CAD build for the part. Positions are in the model's coordinates, mm. Give positions to 0.01 mm unless a question says otherwise; leave off trailing zeros. Loops run counter-clockwise (first coordinate to the right, second up) from the corner with the lowest first, then second, coordinate; pieces in that order, holes last. Notation, with made-up numbers: (14, 28) -> (19, 28) arc R15 cw to (19, 51) -> close; hole circle Ø2 at (62.5, 30.5). An arc over 180 degrees is marked (long way). Use one line per item in the form item = value.
```python
from build123d import *

# Parameters (mm, degrees)
F0_R     = 50
F1_DEPTH = 10
F2_R     = 125
F2_R_2   = 40.44952
F3_DEPTH = 10
F5_DEPTH = 25


with BuildPart() as f1:
    # F0 (on Top) → F1 (new body)
    with BuildSketch(Plane.XY):
        Circle(F0_R)
        Polygon((-10, 30), (0, 30), (10, 30), (10, 10), (30, 10), (30, 0), (30, -10), (10, -10), (10, -30), (0, -30), (-10, -30), (-10, -10), (-30, -10), (-30, 0), (-30, 10), (-10, 10), align=None, mode=Mode.SUBTRACT)
    extrude(amount=F1_DEPTH)

    # F2 (on face) → F3 (join)
    with BuildSketch(Plane.XY.offset(10)):
        Circle(F2_R)
        Circle(F2_R_2, mode=Mode.SUBTRACT)
    extrude(amount=-F3_DEPTH)

    # F4 (on face) → F5 (cut)
    with BuildSketch(Plane.XY.offset(10)):
        with BuildLine():
            Line((0, 116.456337), (0, 104.802647))
            ThreePointArc((0, 104.802647), (9.134153, 104.403842), (18.198789, 103.21046))
            Line((18.198789, 103.21046), (20.222431, 114.687104))
            ThreePointArc((20.222431, 114.687104), (10.149839, 116.013186), (0, 116.456337))
        make_face()
        with BuildLine():
            ThreePointArc((-35.844616, 98.482274), (-27.124921, 101.231584), (-18.198789, 103.21046))
            Line((-18.198789, 103.21046), (-20.222431, 114.687104))
            ThreePointArc((-20.222431, 114.687104), (-30.141118, 112.488184), (-39.830413, 109.433161))
            Line((-39.830413, 109.433161), (-35.844616, 98.482274))
        make_face()
        with BuildLine():
            ThreePointArc((-67.365843, 80.283486), (-60.112329, 85.849303), (-52.401324, 90.761755))
            Line((-52.401324, 90.761755), (-58.228169, 100.854147))
            ThreePointArc((-58.228169, 100.854147), (-66.796611, 95.395447), (-74.856691, 89.21073))
            Line((-74.856691, 89.21073), (-67.365843, 80.283486))
        make_face()
        with BuildLine():
            ThreePointArc((-90.761755, 52.401324), (-85.849303, 60.112329), (-80.283486, 67.365843))
            Line((-80.283486, 67.365843), (-89.21073, 74.856691))
            ThreePointArc((-89.21073, 74.856691), (-95.395447, 66.796611), (-100.854147, 58.228169))
            Line((-100.854147, 58.228169), (-90.761755, 52.401324))
        make_face()
        with BuildLine():
            ThreePointArc((-103.21046, 18.198789), (-101.231584, 27.124921), (-98.482274, 35.844616))
            Line((-98.482274, 35.844616), (-109.433161, 39.830413))
            ThreePointArc((-109.433161, 39.830413), (-112.488184, 30.141118), (-114.687104, 20.222431))
            Line((-114.687104, 20.222431), (-103.21046, 18.198789))
        make_face()
        with BuildLine():
            ThreePointArc((-103.21046, -18.198789), (-104.403842, -9.134153), (-104.802647, 0))
            Line((-104.802647, 0), (-116.456337, 0))
            ThreePointArc((-116.456337, 0), (-116.013186, -10.149839), (-114.687104, -20.222431))
            Line((-114.687104, -20.222431), (-103.21046, -18.198789))
        make_face()
        with BuildLine():
            ThreePointArc((-90.761755, -52.401324), (-94.983455, -44.291513), (-98.482274, -35.844616))
            Line((-98.482274, -35.844616), (-109.433161, -39.830413))
            ThreePointArc((-109.433161, -39.830413), (-105.545285, -49.216575), (-100.854147, -58.228169))
            Line((-100.854147, -58.228169), (-90.761755, -52.401324))
        make_face()
        with BuildLine():
            ThreePointArc((-67.365843, -80.283486), (-74.106663, -74.106663), (-80.283486, -67.365843))
            Line((-80.283486, -67.365843), (-89.21073, -74.856691))
            ThreePointArc((-89.21073, -74.856691), (-82.347066, -82.347066), (-74.856691, -89.21073))
            Line((-74.856691, -89.21073), (-67.365843, -80.283486))
        make_face()
        with BuildLine():
            ThreePointArc((-35.844616, -98.482274), (-44.291513, -94.983455), (-52.401324, -90.761755))
            Line((-52.401324, -90.761755), (-58.228169, -100.854147))
            ThreePointArc((-58.228169, -100.854147), (-49.216575, -105.545285), (-39.830413, -109.433161))
            Line((-39.830413, -109.433161), (-35.844616, -98.482274))
        make_face()
        with BuildLine():
            ThreePointArc((0, -104.802647), (-9.134153, -104.403842), (-18.198789, -103.21046))
            Line((-18.198789, -103.21046), (-20.222431, -114.687104))
            ThreePointArc((-20.222431, -114.687104), (-10.149839, -116.013186), (0, -116.456337))
            Line((0, -116.456337), (0, -104.802647))
        make_face()
        with BuildLine():
            ThreePointArc((35.844616, -98.482274), (27.124921, -101.231584), (18.198789, -103.21046))
            Line((18.198789, -103.21046), (20.222431, -114.687104))
            ThreePointArc((20.222431, -114.687104), (30.141118, -112.488184), (39.830413, -109.433161))
            Line((39.830413, -109.433161), (35.844616, -98.482274))
        make_face()
        with BuildLine():
            ThreePointArc((67.365843, -80.283486), (60.112329, -85.849303), (52.401324, -90.761755))
            Line((52.401324, -90.761755), (58.228169, -100.854147))
            ThreePointArc((58.228169, -100.854147), (66.796611, -95.395447), (74.856691, -89.21073))
            Line((74.856691, -89.21073), (67.365843, -80.283486))
        make_face()
        with BuildLine():
            ThreePointArc((90.761755, -52.401324), (85.849303, -60.112329), (80.283486, -67.365843))
            Line((80.283486, -67.365843), (89.21073, -74.856691))
            ThreePointArc((89.21073, -74.856691), (95.395447, -66.796611), (100.854147, -58.228169))
            Line((100.854147, -58.228169), (90.761755, -52.401324))
        make_face()
        with BuildLine():
            ThreePointArc((103.21046, -18.198789), (101.231584, -27.124921), (98.482274, -35.844616))
            Line((98.482274, -35.844616), (109.433161, -39.830413))
            ThreePointArc((109.433161, -39.830413), (112.488184, -30.141118), (114.687104, -20.222431))
            Line((114.687104, -20.222431), (103.21046, -18.198789))
        make_face()
        with BuildLine():
            ThreePointArc((103.21046, 18.198789), (104.403842, 9.134153), (104.802647, 0))
            Line((104.802647, 0), (116.456337, 0))
            ThreePointArc((116.456337, 0), (116.013186, 10.149839), (114.687104, 20.222431))
            Line((114.687104, 20.222431), (103.21046, 18.198789))
        make_face()
        with BuildLine():
            ThreePointArc((90.761755, 52.401324), (94.983455, 44.291513), (98.482274, 35.844616))
            Line((98.482274, 35.844616), (109.433161, 39.830413))
            ThreePointArc((109.433161, 39.830413), (105.545285, 49.216575), (100.854147, 58.228169))
            Line((100.854147, 58.228169), (90.761755, 52.401324))
        make_face()
        with BuildLine():
            ThreePointArc((67.365843, 80.283486), (74.106663, 74.106663), (80.283486, 67.365843))
            Line((80.283486, 67.365843), (89.21073, 74.856691))
            ThreePointArc((89.21073, 74.856691), (82.347066, 82.347066), (74.856691, 89.21073))
            Line((74.856691, 89.21073), (67.365843, 80.283486))
        make_face()
        with BuildLine():
            ThreePointArc((35.844616, 98.482274), (44.291513, 94.983455), (52.401324, 90.761755))
            Line((52.401324, 90.761755), (58.228169, 100.854147))
            ThreePointArc((58.228169, 100.854147), (49.216575, 105.545285), (39.830413, 109.433161))
            Line((39.830413, 109.433161), (35.844616, 98.482274))
        make_face()
    extrude(amount=-F5_DEPTH, mode=Mode.SUBTRACT)


solid = f1.part
```
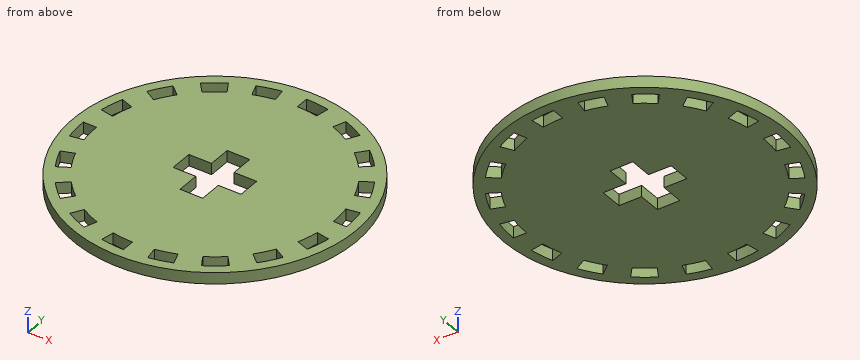
1. Cut at D-D, the plane x = 13. Write the cut outline in (y, z).
Result sheet:
outline = (-124.32, 0) -> (-10, 0) -> (-10, 10) -> (-124.32, 10) -> close; (10, 0) -> (103.99, 0) -> (103.99, 10) -> (10, 10) -> close; (115.73, 0) -> (124.32, 0) -> (124.32, 10) -> (115.73, 10) -> close
2. Drop flat-ended pins along their axis: P1, Ø5, axis at x = 23, z = 3.5, coming from the +Y side; P2, Ø2, axis at x = 29, z = 5, coming from the -Y side; P3, Ø6, axis at y = -45.5, z = 7, coming from the -X side. Give the stop position or say it passes through.
Result sheet:
P1 = 123.31
P2 = -121.82
P3 = -117.55
3. Drill centre lines: line 1 (X direction, y = 55.5, z = 2); line 2 (Y direction, x = 14, z = 5.5); line 3 (Y direction, x = -4, z = 4.5). Where is each one in solid material? Low to high.
Result sheet:
line_1 = -112 to -96.13, -88.9 to 96.13, 102.38 to 112
line_2 = -124.21 to -10, 10 to 103.86, 115.61 to 124.21
line_3 = -124.94 to -116.39, -104.73 to -30, 30 to 124.94
4. Cut at C-C, the plane z = 5.5. State how many separate pieces and enclosed holes the cut face has, then the cut area to 3 significant figures.
Result sheet:
separate_pieces = 1
enclosed_holes = 19
area = 43,000 mm^2
5. Cut at B-B, the plane x = -43. Write the cut outline in (y, z), then the cut area to 3 significant figures.
Result sheet:
outline = (-117.37, 0) -> (-108.23, 0) -> (-108.23, 10) -> (-117.37, 10) -> close; (-95.58, 0) -> (117.37, 0) -> (117.37, 10) -> (-95.58, 10) -> close
area = 2,220 mm^2
6. Cut at A-A, the plane x = -94. Write the cut outline in (y, z), then the cut area to 3 significant figures.
Result sheet:
outline = (-82.4, 0) -> (-54.27, 0) -> (-54.27, 10) -> (-82.4, 10) -> close; (-46.34, 0) -> (54.27, 0) -> (54.27, 10) -> (-46.34, 10) -> close; (68.75, 0) -> (82.4, 0) -> (82.4, 10) -> (68.75, 10) -> close
area = 1,420 mm^2
